Part model, mm, in its own coordinate system. Coordinates: 2 decimals unless noted, no trailing zeros. Loops run counter-clockwise (first coordinate to the right, second up) from the corner with the lowest first, then second, coordinate; pieces in that order, holes last. Notation, with made-up numbers: M 83,-34 L 101,-34 A13 ccw 101,-22 Z; hole C 50.25,0.5 d1. An arc over 180 degrees is marked long. Answer as a JSON object with one key per item and string values. Group by question number.
1. Saw through at C-C on x = 8.75. Write the cut outline in (y, z), then the cut area to 3 significant figures.
2. Saw through at A-A on z = -55.5. Write the cut outline in (x, y).
3. Mould opens along X. For faces 1 (the face through (13.044, 2.248, -1.513)), 2 (the face through (9, 5, -100)), 3 (the face through (13.25, 2.07, -95.42)) say: released by +X, released by -X, zero draft, split by the parting line, or undercut.
4. Saw through at B-B on x = 1. Write the cut outline in (y, z).
5. Drill centre lines: L1, parallel to Z at x = 13.5, y = 2.5; L2, parallel to X at y = -1.5, z = -8.5; L3, parallel to Y at x = 15.75, z = -85. Where is each one in solid material? Low to high.
6. Drop flat-ended pins along their axis: pin 1 Ø4 at (x, z) = (13, -79.5) entering from -Y; pin 2 Ø1.5 at (x, z) = (5, -83) entering from -Y; pin 3 Ø1.5 at (x, z) = (13.5, -27) entering from -Y; pin 4 Ø5 at (x, y) = (4, 3.5) entering from -Z (3 decimals). Give the stop position or say it passes through.
Autodesk Inventor part; units mm, degrees
ref_plane "Work Plane2" through (40.3431, -2.6133, -6) normal (0, -1, 0) x (1, 0, 0)
ref_plane "Płaszczyzna konstrukcyjna3" through (19.0877, -1.5003, -6) normal (0, -1, 0) x (1, 0, 0)
ref_plane "YZ Plane" through (0, 0, 0) normal (1, 0, 0) x (0, 1, 0)
sketch "Sketch1" plane through (0, 0, 0) normal (0, 0, 1) x (1, 0, 0)
  line L0 (10.7451, 5.5) -> (50.1922, -27.6)
  line L1 (50.1922, -27.6) -> (100, -27.6)
  line L2 (100, -27.6) -> (100, -23.6)
  line L3 (100, -23.6) -> (83.9, -23.6)
  arc A0 (65.8, -5.5) -> (83.9, -23.6) centre (83.9, -5.5) ccw
  line L4 (65.8, -5.5) -> (65.8, 5.5)
  line L5 (65.8, 5.5) -> (10.7451, 5.5)
  line L6 (7.1699, 8.5) -> (10.7451, 5.5)
  line L7 (65.8, 5.5) -> (10.7451, 5.5)
  line L8 (65.8, 5.5) -> (65.8, 8.5)
  line L9 (65.8, 8.5) -> (7.1699, 8.5)
  circle A1 centre (83.9, -5.5) radius 16.1
  line L10 (83.9, 10.6) -> (-17.1951, 10.6)
  line L11 (100, -5.5) -> (0, -5.5)
  line L12 (0, -5.5) -> (0, 10.6)
  line L13 (7.1699, 8.5) -> (4.6672, 10.6)
  line L14 (7.1699, 8.5) -> (5.2415, 6.2019)
  line L15 (5.2415, 6.2019) -> (0, 10.6)
  line L16 (0, 10.6) -> (22.9813, -8.6836)
  line L17 (22.9813, -8.6836) -> (24.9097, -6.3855)
  point P0 (0, 0)
  dimension "d0" = 100
  dimension "d1" = 3
  dimension "d2" = 30
extrude "Extrusion1" add sketch "Sketch1" against normal blind 100 contours L17 L16 L11 L0 | L11 L16 L14 L6 L0 | L14 L15 L10 L13
ref_plane "Work Plane1" through (8.1777, -6.0133, 8.6215) normal (0, -1, 0) x (0, 0, 1)
sketch "Sketch2" plane through (8.1777, -6.0133, 8.6215) normal (0, -1, 0) x (0, 0, 1)
  line L0 (-22.0032, -27.7487) -> (35.8312, 20.7819)
  line L1 (35.8312, 20.7819) -> (3.0626, 38.2053)
  line L2 (3.0626, 38.2053) -> (-26.1922, -24.5344)
  line L3 (-26.1922, -24.5344) -> (-22.0032, -27.7487)
  line L4 (-46.8404, -23.7111) -> (-15.3118, 43.9022)
  line L5 (-15.3118, 43.9022) -> (-51.9953, 38.492)
  line L6 (-51.9953, 38.492) -> (-51.9953, -22.5683)
  line L7 (-51.9953, -22.5683) -> (-46.8404, -23.7111)
  line L8 (-70.2281, -23.6979) -> (-65.0733, -22.5551)
  line L9 (-65.0733, -22.5551) -> (-65.0733, 38.4893)
  line L10 (-94.9551, 29.3293) -> (-70.2281, -23.6979)
  line L11 (-65.0733, 38.4893) -> (-94.9551, 29.3293)
  line L12 (-90.9709, -24.4596) -> (-115.5317, 28.2112)
  arc A0 (-115.5317, 28.2112) -> (-139.4308, 9.4739) centre (-87.2125, -32.5195) ccw
  line L13 (-139.4308, 9.4739) -> (-95.1598, -27.6739)
  line L14 (-95.1598, -27.6739) -> (-90.9709, -24.4596)
  point P0 (-8.6215, 8.1777)
  point P1 (-24.0977, -26.1415)
  point P2 (-49.4178, -23.1397)
  point P3 (-67.6507, -23.1265)
  point P4 (-93.0654, -26.0667)
ref_plane "Work Plane2" through (40.3431, -2.6133, -6) normal (0, -1, 0) x (1, 0, 0)
extrude "Extrusion2" cut sketch "Sketch2" against normal up to surface (3.4 mm away)
extrude "Extrusion3" cut sketch "Sketch2" along normal blind 1
sketch "Sketch3" plane through (15.747, -2.6133, 0) normal (0, -1, 0) x (1, 0, 0)
  line L0 (4.6672, 0) -> (4.6672, -11.8362)
  line L1 (0, 0) -> (4.6672, 0)
  line L2 (0, -9.66) -> (0, 0)
  line L3 (4.6672, -11.8362) -> (0, -9.66)
  line L4 (4.6672, -32.8682) -> (4.6672, -43.3737)
  line L5 (0, -30.6918) -> (4.6672, -32.8682)
  line L6 (0, -43.3737) -> (0, -30.6918)
  line L7 (4.6672, -43.3737) -> (0, -43.3737)
  line L8 (4.6672, -56.4518) -> (4.6672, -66.9512)
  line L9 (0, -56.4518) -> (4.6672, -56.4518)
  line L10 (0, -69.1275) -> (0, -56.4518)
  line L11 (4.6672, -66.9512) -> (0, -69.1275)
  line L12 (4.6672, -88.0491) -> (4.6672, -100)
  line L13 (0, -90.2254) -> (4.6672, -88.0491)
  line L14 (0, -100) -> (0, -90.2254)
  line L15 (4.6672, -100) -> (0, -100)
  line L16 (0, -90.2254) -> (12.0968, -84.5846)
  line L17 (0, -90.2254) -> (4.6672, -88.0491)
  line L18 (12.0968, -84.5846) -> (12.0968, -100)
  line L19 (4.6672, -100) -> (0, -100)
  line L20 (12.0968, -100) -> (0, -100)
  line L21 (8.636, -100) -> (8.636, -86.1984)
  line L22 (8.636, -86.1984) -> (9.1627, -85.9528)
  line L23 (9.1627, -64.8548) -> (9.1627, -85.9528)
  line L24 (9.1627, -64.8548) -> (8.636, -65.1005)
  line L25 (8.636, -65.1005) -> (8.636, -56.4518)
  line L26 (8.636, -56.4518) -> (9.1627, -56.4518)
  line L27 (9.1627, -43.3737) -> (9.1627, -56.4518)
  line L28 (9.1627, -43.3737) -> (8.636, -43.3737)
  line L29 (8.636, -43.3737) -> (8.636, -34.7188)
  line L30 (8.636, -34.7188) -> (9.1627, -34.9645)
  line L31 (9.1627, -13.9325) -> (9.1627, -34.9645)
  line L32 (9.1627, -13.9325) -> (8.636, -13.6868)
  line L33 (8.636, -13.6868) -> (8.636, 0)
  line L34 (7.2344, 0) -> (8.636, 0)
  line L35 (7.2344, 0) -> (7.2344, -100)
  line L36 (8.636, -100) -> (7.2344, -100)
  line L37 (0, -30.6918) -> (5.2437, -33.137)
  line L38 (5.2437, -33.137) -> (5.2437, -43.3737)
  line L39 (5.2437, -43.3737) -> (0, -43.3737)
  line L40 (0, -43.3737) -> (0, -30.6918)
  line L41 (5.2437, -66.6823) -> (0, -69.1275)
  line L42 (0, -69.1275) -> (0, -56.4518)
  line L43 (0, -56.4518) -> (5.2437, -56.4518)
  line L44 (5.2437, -56.4518) -> (5.2437, -66.6823)
  line L45 (5.2437, -87.7803) -> (5.2437, -100)
  line L46 (7.2344, -100) -> (5.2437, -100)
  line L47 (7.2344, 0) -> (7.2344, -100)
  line L48 (5.2437, 0) -> (7.2344, 0)
  line L49 (5.2437, 0) -> (5.2437, -12.1051)
  line L50 (5.2437, -12.1051) -> (0, -9.66)
  line L51 (0, -9.66) -> (0, 0)
  line L52 (-15.747, 0) -> (0, 0)
  line L53 (-15.747, 0) -> (-15.747, -100)
  line L54 (0, -100) -> (-15.747, -100)
  line L55 (0, -100) -> (0, -90.2254)
  line L56 (0, -90.2254) -> (5.2437, -87.7803)
  line L57 (4.6672, -66.9512) -> (0, -69.1275)
  line L58 (0, -69.1275) -> (9.1627, -64.8548)
  line L59 (9.1627, -56.4518) -> (4.6672, -56.4518)
  line L60 (9.1627, -56.4518) -> (9.1627, -64.8548)
  line L61 (0, -56.4518) -> (9.1627, -56.4518)
  line L62 (0, -43.3737) -> (9.1627, -43.3737)
  line L63 (8.636, -34.7188) -> (9.1627, -34.9645)
  line L64 (9.1627, -34.9645) -> (9.1627, -43.3737)
  line L65 (8.636, -43.3737) -> (8.636, -34.7188)
  line L66 (0, -30.6918) -> (4.6672, -32.8682)
  line L67 (0, -30.6918) -> (9.1627, -34.9645)
  line L68 (4.6672, -11.8362) -> (0, -9.66)
  line L69 (4.6672, -11.8362) -> (9.1627, -13.9325)
  line L70 (9.1627, -13.9325) -> (9.1627, 0)
  line L71 (9.1627, 0) -> (0, 0)
  line L72 (4.6672, 0) -> (-11.0798, 0)
  line L73 (8.9504, 0) -> (9.1627, -0.253)
  line L74 (9.1627, 0) -> (9.1627, -0.253)
  line L75 (8.9504, 0) -> (9.1627, 0)
  line L76 (9.1627, -99.5783) -> (8.8088, -100)
  line L77 (9.1627, -100) -> (8.8088, -100)
  line L78 (9.1627, -99.5783) -> (9.1627, -100)
  point P0 (-15.747, 0)
  point P1 (8.9504, 0)
  point P2 (5.2437, -12.1051)
  point P3 (7.2344, 0)
  point P4 (5.2437, -33.137)
  point P5 (5.2437, -43.3737)
  point P6 (5.2437, -66.6823)
  point P7 (5.2437, -87.7803)
  point P8 (5.2437, -100)
  point P9 (8.636, -100)
  point P10 (8.636, -86.1984)
extrude "Extrusion4" cut sketch "Sketch3" along normal through all contours L48 L35 L69 L49 | L34 L33 L69 L35 | L67 L29 L62 L35 | L35 L62 L38 L67 | L71 L70 L73 | L59 L25 L58 L35 | L35 L58 L44 L59 | L45 L16 L35 L20 | L16 L21 L20 L35 | L76 L78 L20
sketch "Sketch4" plane through (0, 10.6, -100) normal (-0.6427876, -0.7660444, 0) x (0.7660444, -0.6427876, 0)
  line L0 (30, 34.2459) -> (20.5562, 30.8725)
  line L1 (20.5562, 30.8725) -> (20.5562, 43.5482)
  line L2 (20.5562, 43.5482) -> (30, 43.5482)
  line L3 (30, 56.6263) -> (30, 43.5482)
  line L4 (30, 56.6263) -> (20.5562, 56.6263)
  line L5 (20.5562, 56.6263) -> (20.5562, 69.3082)
  line L6 (20.5562, 69.3082) -> (30, 65.9347)
  line L7 (30, 86.9667) -> (30, 65.9347)
  line L8 (30, 86.9667) -> (20.5562, 90.34)
  line L9 (20.5562, 90.34) -> (20.5562, 100)
  line L10 (0, 100) -> (20.5562, 100)
  line L11 (0, 100) -> (0, 0)
  line L12 (20.5562, 0) -> (0, 0)
  line L13 (20.5562, 0) -> (20.5562, 9.7746)
  line L14 (20.5562, 9.7746) -> (30, 13.148)
  line L15 (30, 34.2459) -> (30, 13.148)
  line L16 (73.894, 94) -> (30.9766, 94)
  line L17 (24.1315, 94) -> (11.5095, 94)
  line L18 (31.2695, 94) -> (24.1315, 94)
  line L19 (0, 100) -> (0, 0)
  line L20 (0, 50) -> (30, 50.0873)
  line L21 (20.5562, 100) -> (18.5562, 100)
  line L22 (18.5562, 100) -> (18.5562, 94)
  line L23 (18.5562, 94) -> (20.5562, 94)
  line L24 (20.5562, 94) -> (20.5562, 100)
  circle A0 centre (15.5562, 97) radius 3
  circle A1 centre (15.5562, 97) radius 1.5
  circle A2 centre (15.8294, 3.0913) radius 1.5
  point P0 (6.8135, 100)
  dimension "d11" = 2
  dimension "d12" = 3
extrude "Extrusion5" cut sketch "Sketch4" against normal blind 10 contours A1 | A2
chamfer "Chamfer1" distance 1 angle 45 2 edges at (10.9769, 1.3893, -96.9087) (10.7677, 1.5648, -3)
sketch "Szkic5" plane through (15.747, -2.6133, 0) normal (0, -1, 0) x (1, 0, 0)
  line L0 (4.6672, 0) -> (4.6672, -11.8362)
  line L1 (0, 0) -> (4.6672, 0)
  line L2 (0, -9.66) -> (0, 0)
  line L3 (4.6672, -11.8362) -> (0, -9.66)
  line L4 (4.6672, -32.8682) -> (4.6672, -43.3737)
  line L5 (0, -30.6918) -> (4.6672, -32.8682)
  line L6 (0, -43.3737) -> (0, -30.6918)
  line L7 (4.6672, -43.3737) -> (0, -43.3737)
  line L8 (4.6672, -56.4518) -> (4.6672, -66.9512)
  line L9 (0, -56.4518) -> (4.6672, -56.4518)
  line L10 (0, -69.1275) -> (0, -56.4518)
  line L11 (4.6672, -66.9512) -> (0, -69.1275)
  line L12 (4.6672, -88.0491) -> (4.6672, -100)
  line L13 (0, -90.2254) -> (4.6672, -88.0491)
  line L14 (0, -100) -> (0, -90.2254)
  line L15 (4.6672, -100) -> (0, -100)
  line L16 (4.6672, 0) -> (4.6672, -11.8362)
  line L17 (4.6672, 0) -> (-31.1129, 0)
  line L18 (-31.1129, 0) -> (-31.1129, -100)
  line L19 (-31.1129, -100) -> (4.6672, -100)
  line L20 (4.6672, -100) -> (4.6672, 0)
  line L21 (4.6672, -100) -> (0, -100)
  line L22 (4.6672, 0) -> (-11.0798, 0)
  line L23 (4.6672, 0) -> (18.0688, 0)
  line L24 (18.0688, 0) -> (18.0688, -100)
  line L25 (18.0688, -100) -> (4.6672, -100)
  line L26 (4.6672, -100) -> (4.6672, 0)
  point P0 (-15.747, 0)
  point P1 (4.6672, -100)
extrude "Wyciągnięcie proste6" cut sketch "Szkic5" along normal blind 10
ref_plane "Płaszczyzna konstrukcyjna3" through (19.0877, -1.5003, -6) normal (0, -1, 0) x (1, 0, 0)
extrude "Wyciągnięcie proste7" cut sketch "Szkic5" against normal up to surface (1.113 mm away)
sketch "Szkic6" plane through (0, 0, 0) normal (0, 0, 1) x (1, 0, 0)
  line L0 (14.4205, -1.5003) -> (19.0877, -1.5003)
  line L1 (19.0877, -1.5003) -> (4.6672, 10.6)
  line L2 (4.6672, 10.6) -> (0, 10.6)
  line L3 (0, 10.6) -> (14.4205, -1.5003)
  line L4 (0, 10.6) -> (15.3209, -2.2558)
  line L5 (15.3209, -2.2558) -> (17.2493, 0.0424)
  line L6 (19.0877, -1.5003) -> (4.6672, 10.6)
  point P0 (0, 0)
  point P1 (15.9548, -1.5003)
  dimension "d22" = 20
extrude "Wyciągnięcie proste8" cut sketch "Szkic6" against normal through all contours L5 L1 L0
extrude "Wyciągnięcie proste9" add sketch "Szkic6" against normal up to surface (100 mm away) contours L0 L5 L4
properties part number "strug" material "Steel, Alloy"
Outcome:
{
 "1": {"outline": "M 3.26,-100 L 7.17,-100 L 7.17,0 L 3.26,0 Z", "area": "392 mm²"},
 "2": {"outline": "M 0,10.6 L 5.24,6.2 L 14.42,-1.5 L 15.32,-2.26 L 17.25,0.04 L 10.75,5.5 L 7.17,8.5 L 4.67,10.6 Z"},
 "3": {"face 1": "undercut", "face 2": "zero draft", "face 3": "undercut"},
 "4": {"outline": "M 9.76,-100 L 10.6,-100 L 10.6,0 L 9.76,0 Z"},
 "5": {"L1": "z = -100 to -98.38, -95.44 to -4.5, -1.5 to 0", "L2": "x = 14.42 to 15.96", "L3": "y = -1.74 to 1.3"},
 "6": {"pin 1": "stops at y = -1.99", "pin 2": "stops at y = 5.78", "pin 3": "stops at y = -1.36", "pin 4": "passes through"}
}
